Design review of the part built by this model. Coordinates are the model's own, in mm. Face numbers are marked on the shaded views. Give positions to 0.01 mm unless a question says otherwise; leave off trailing zeros. Write each loop counter-clockwise with the first axis right and the second up, starting at its lowest first coordinate (ties: lowest second). Pieces come first, ordered by that corner, then holes. Notation, with made-up numbers: (16.25, 31) -> (22.25, 31) arc R25 cw to (22.25, 43) -> close; hole circle Ø5 at (-5, 89). An arc over 180 degrees is marked (long way). Return JSON: item names as keys, results as strings. Group by question number.
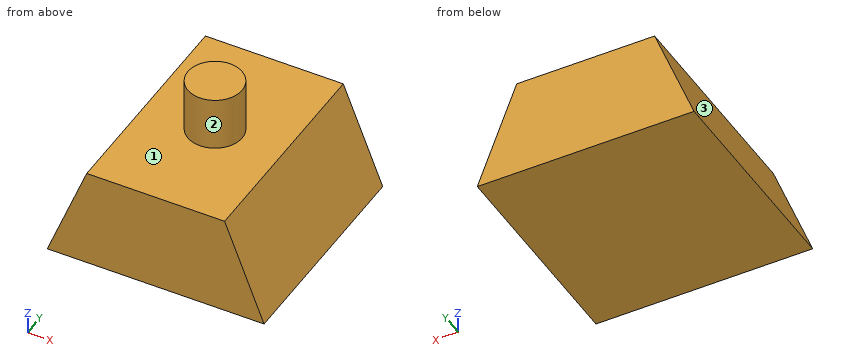
from build123d import *

# Parameters (mm, degrees)
F1_DEPTH = 20
F2_R     = 2.5
F3_DEPTH = 5


with BuildPart() as f1:
    # F0 (on Front) → F1 (new body)
    with BuildSketch(Plane.XZ):
        Polygon((6.36, 0), (0, 0), (-6.36, 0), (-10, -9.313989), (0, -9.313989), (10, -9.313989), align=None)
    extrude(amount=F1_DEPTH)

    # F2 (on face) → F3 (join)
    with BuildSketch(Plane.XY):
        with Locations((0, -10)):
            Circle(F2_R)
    extrude(amount=F3_DEPTH)


solid = f1.part
Q1. For L1, parallel to Z at x = -4.75, y = -3; L2, parallel to Y at x = 0, z = 2; L3, parallel to X at y = -7, z = -7.5, list the stretches that pass through material, from the lowest coordinate up. Write a range as from..to.
Q2. Take a section at C-C, the plane z = 1. Give the boundary of the cut face in (x, y).
Q3. Take a section at B-B, the plane x = 0. Give the boundary of the cut face in (y, z).
Q4. Take a section at D-D, the plane y = -7. Give the boundary of the cut face in (x, z).
Q5. Insertion check: pin 1 (6 mm diameter, centred on y = -7, z = -0.5, fed in from +X); pin 2 (3 mm diameter, centred on x = -0.5, z = 2, fed in from -Y). Each pin has a flat end and moves straight along its axis. Give the tip position at first contact, or say it passes through.
Q6. Mouldability with a two-part tool opening along X and no side actions: class the marked faces 1, 2 and 3 as +X half, -X half, draft (parallel to the pull), parting line (faces both ways), or undercut.
Q7. Take a section at A-A, the plane y = -10. Give the boundary of the cut face in (x, z).
Final values:
{
 "1": {"L1": "z = -9.31..0", "L2": "y = -12.5..-7.5", "L3": "x = -9.29..9.29"},
 "2": {"outline": "circle Ø5 at (0, -10)"},
 "3": {"outline": "(-20, -9.31) -> (0, -9.31) -> (0, 0) -> (-7.5, 0) -> (-7.5, 5) -> (-12.5, 5) -> (-12.5, 0) -> (-20, 0) -> close"},
 "4": {"outline": "(-10, -9.31) -> (10, -9.31) -> (6.36, 0) -> (-6.36, 0) -> close"},
 "5": {"pin 1": "stops at x = 7.73", "pin 2": "stops at y = -12.5"},
 "6": {"face 1": "draft", "face 2": "parting line", "face 3": "-X half"},
 "7": {"outline": "(-10, -9.31) -> (10, -9.31) -> (6.36, 0) -> (2.5, 0) -> (2.5, 5) -> (-2.5, 5) -> (-2.5, 0) -> (-6.36, 0) -> close"}
}
